Here's how the part is built. I have some questions about the finished solid (model axes, mm). Round coordinates to 2 decimals unless told otherwise and drop trailing zeros. Order: outer loops, then holes, each group sorted by start corner. A loop starts at its lowest first (then second) coordinate and runs counter-clockwise, first axis right, second up. Notation, with made-up numbers: (-33, -9.5) -> (-5, -9.5) arc R28 ccw to (-5, 21.5) -> close; hole circle Ø11 at (33, 53.5). An arc over 180 degrees is marked (long way). One line per item, written item: value.
```python
from build123d import *

# Parameters (mm, degrees)
SKETCH1_R           = 1.5
BOSS_EXTRUDE1_DEPTH = 4
FILLET1_R           = 0.2
SKETCH2_W           = 2.5
SKETCH2_H           = 2
CUT_EXTRUDE1_DEPTH  = 1
FILLET3_R           = 0.1
FILLET4_R           = 0.2
FILLET5_R           = 0.5


with BuildPart() as part:
    # Sketch1 → Boss-Extrude1 (new body)
    with BuildSketch(Plane(origin=(0, 0, 0), x_dir=(1, 0, 0), z_dir=(0, 1, 0))):
        with Locations(Location((0, 0, 0), (0, 0, 270))):
            Circle(SKETCH1_R)
    extrude(amount=BOSS_EXTRUDE1_DEPTH)

    # Fillet1
    fillet1_edges = [part.edges().sort_by_distance(p)[0] for p in [
        (0, 0, -1.5),
    ]]
    fillet(fillet1_edges, radius=FILLET1_R)

    # Sketch2 → Revolve1 (revolve)
    with BuildSketch(Plane.XY, mode=Mode.PRIVATE) as revolve1_sk:
        with Locations((-1.25, 5)):
            Rectangle(SKETCH2_W, SKETCH2_H)
    revolve(revolve1_sk.sketch.rotate(Axis((0, 0, 0), (0, 1, 0)), 270), axis=Axis((0, 0, 0), (0, 1, 0)))

    # Sketch3 → Cut-Extrude1 (cut)
    with BuildSketch(Plane(origin=(0, 6, 0), x_dir=(1, 0, 0), z_dir=(0, 1, 0))):
        Polygon((-0.5, 0.5), (-1.5, 0.5), (-1.5, -0.5), (-0.5, -0.5), (-0.5, -1.5), (0.5, -1.5), (0.5, -0.5), (1.5, -0.5), (1.5, 0.5), (0.5, 0.5), (0.5, 1.5), (-0.5, 1.5), align=None)
    extrude(amount=-CUT_EXTRUDE1_DEPTH, mode=Mode.SUBTRACT)

    # Fillet3
    fillet3_edges = [part.edges().sort_by_distance(p)[0] for p in [
        (0.5, 6, 1),
        (1, 6, 0.5),
        (1.5, 6, 0),
        (1, 6, -0.5),
        (0.5, 6, -1),
        (0, 6, -1.5),
        (-0.5, 6, -1),
        (-1, 6, -0.5),
        (-1.5, 6, 0),
        (-1, 6, 0.5),
        (-0.5, 6, 1),
        (0, 6, 1.5),
    ]]
    fillet(fillet3_edges, radius=FILLET3_R)

    # Fillet4
    fillet4_edges = [part.edges().sort_by_distance(p)[0] for p in [
        (0.5, 5, 1),
        (0, 5, 1.5),
        (-0.5, 5, 1),
        (-1, 5, 0.5),
        (-1.5, 5, 0),
        (-1, 5, -0.5),
        (-0.5, 5, -1),
        (0, 5, -1.5),
        (0.5, 5, -1),
        (1, 5, -0.5),
        (1.5, 5, 0),
        (1, 5, 0.5),
    ]]
    fillet(fillet4_edges, radius=FILLET4_R)

    # Fillet5
    fillet5_edges = [part.edges().sort_by_distance(p)[0] for p in [
        (0, 6, 2.5),
    ]]
    fillet(fillet5_edges, radius=FILLET5_R)


solid = part.part
```
Q1. I want a section at A-A on z = 0. Write out the boundary of the cut face in (x, y), then the cut area to 3 significant figures.
Answers:
outline: (-2.5, 4) -> (-1.5, 4) -> (-1.5, 0.2) arc R0.2 ccw to (-1.3, 0) -> (1.3, 0) arc R0.2 ccw to (1.5, 0.2) -> (1.5, 4) -> (2.5, 4) -> (2.5, 5.5) arc R0.5 ccw to (2, 6) -> (1.6, 6) arc R0.1 ccw to (1.5, 5.9) -> (1.5, 5.2) arc R0.2 cw to (1.3, 5) -> (-1.3, 5) arc R0.2 cw to (-1.5, 5.2) -> (-1.5, 5.9) arc R0.1 ccw to (-1.6, 6) -> (-2, 6) arc R0.5 ccw to (-2.5, 5.5) -> close
area: 18.9 mm2
Q2. I want a section at B-B on x = 0. Write out the boundary of the cut face in (y, z).
Answers:
outline: (0, -1.3) arc R0.2 ccw to (0.2, -1.5) -> (4, -1.5) -> (4, -2.5) -> (5.5, -2.5) arc R0.5 ccw to (6, -2) -> (6, -1.6) arc R0.1 ccw to (5.9, -1.5) -> (5.2, -1.5) arc R0.2 cw to (5, -1.3) -> (5, 1.3) arc R0.2 cw to (5.2, 1.5) -> (5.9, 1.5) arc R0.1 ccw to (6, 1.6) -> (6, 2) arc R0.5 ccw to (5.5, 2.5) -> (4, 2.5) -> (4, 1.5) -> (0.2, 1.5) arc R0.2 ccw to (0, 1.3) -> close
Q3. I need wall thicknesses on line 1 along Y through (x, z) = (-0.15, -0.1); line 2 along Z through (x, y) = (-0.35, 5.7); line 3 along Y through (x, z) = (0.05, 1.6). Which ranges of each line are inside material? Lowest first, please.
Answers:
line 1: 0 to 5
line 2: -2.43 to -1.5, 1.5 to 2.43
line 3: 4 to 6
Q4. I want a section at D-D on y = 1.4. Write out the boundary of the cut face in (x, z), then the cut area to 3 significant figures.
Answers:
outline: circle Ø3 at (0, 0)
area: 7.07 mm2
Q5. For P1, Ø0.8, axis at y = 5.5, z = -1, coming from the +X side; P2, Ø2, axis at x = -2, y = 4, coming from the +Z side; P3, Ø0.8, axis at x = -1, y = 5.5, coming from the +Z side, each with a flat end and sliding along its axis, tell me the tip position at first contact or that it passes through.
Answers:
P1: x = 2.43
P2: z = 2.29
P3: z = 2.43
Q6. If we mould it in two halves opening along Z, with no side actions, what happens to faces 1 (the face through (2, 4, 0)), 2 (the face through (0, 5, 0)), 3 (the face through (0.45, 2.07, 1.43))? For each: pulls with the +Z half, pulls with the -Z half, needs draft (parallel to the pull), parting line crosses it, or undercut.
Answers:
face 1: needs draft
face 2: undercut
face 3: parting line crosses it
Q7. I want a section at C-C on y = 4.35. Write out the boundary of the cut face in (x, z), then the cut area to 3 significant figures.
Answers:
outline: circle Ø5 at (0, 0)
area: 19.6 mm2
